Autodesk Inventor part; units mm, degrees
ref_plane "YZ Plane" through (0, 0, 0) normal (1, 0, 0) x (0, 1, 0)
ref_plane "XZ Plane" through (0, 0, 0) normal (0, 1, 0) x (-1, 0, 0)
ref_plane "XY Plane" through (0, 0, 0) normal (0, 0, 1) x (1, 0, 0)
sketch "Sketch1" plane through (0, 0, 0) normal (0, 1, 0) x (-1, 0, 0)
  line L0 (81, 0) -> (0, 0)
  line L1 (0, 0) -> (0, -32)
  line L2 (0, -32) -> (81, -32)
  line L3 (81, -32) -> (81, 0)
  point P0 (0, -16)
  point P1 (40.5, 0)
  dimension "d0" = 81
  dimension "d1" = 32
extrude "Extrusion1" add sketch "Sketch1" along normal blind 20
sketch "Sketch2" plane through (0, 0, 0) normal (1, 0, 0) x (0, 0, -1)
  line L0 (0, 0) -> (32, 0)
  line L1 (24.1, 0) -> (24.1, 6.35)
  line L2 (24.1, 6.35) -> (25.6, 6.35)
  line L3 (25.6, 6.35) -> (25.6, 9.525)
  line L4 (25.6, 9.525) -> (6.4, 9.525)
  line L5 (6.4, 9.525) -> (6.4, 6.35)
  line L6 (6.4, 6.35) -> (7.9, 6.35)
  line L7 (7.9, 6.35) -> (7.9, 0)
  line L8 (24.1, 0) -> (7.9, 0)
  line L9 (32, 0) -> (32, 20)
  line L10 (0, 0) -> (0, 20)
  dimension "d4" = 3.175
  dimension "d5" = 6.35
  dimension "d6" = 19.2
  dimension "d7" = 16.2
  dimension "d8" = 6.4
  dimension "d17" = 7.9
  dimension "d18" = 32
extrude "Extrusion2" cut sketch "Sketch2" against normal blind 103.1875
fillet "Fillet1" radius 2 1 edges at (-40.5, 20, -32)
fillet "Fillet2" radius 2 1 edges at (-40.5, 20, 0)
equation "\"d8\" = -0.5 * d6 + 0.5 * d18"
equation "\"d17\" = -0.5 * d7 + 0.5 * d18"
properties part number "rail holder"
Can you work these out from the model? Positions are in its coordinate system, mm. A direction names the side the tool comes from. Round coordinates to 2 decimals unless told otherwise and drop trailing zeros. Loops run counter-clockwise (first coordinate to the right, second up) from the corner with the lowest first, then second, coordinate; pieces in that order, holes last. Notation, with made-up numbers: M 13,67.25 L 23,67.25 A15 ccw 23,73.25 Z; hole C 68,27 d7. An arc over 180 degrees is marked long. Answer in a Markdown table with one row per item.
1. On a 3-axis mill with a long thin cutter (end or side, diameter ignored), from which of +Z, -Z, +X, -X, +Y, -Y can I reach the whole of each face in a straight line? I mean faces 1 (the face through (-40, 6.35, -7)), 2 (the face through (-40, 3, -7.9)), 3 (the face through (-41.07, 19.43, -31.4)). Say none if no direction works.
Established:
| item | result |
|---|---|
| face 1 | +X, -X |
| face 2 | +X, -X, -Y |
| face 3 | -Z, +X, -X, +Y |
2. If we section it at C-C, the plane z = -22: Please give me the cut outline in (x, y) (3 decimals).
Established:
| item | result |
|---|---|
| outline | M -81,9.525 L 0,9.525 L 0,20 L -81,20 Z |
3. Thinking about a two-plate mould opening in Y: for faces 4 (the face through (-40, 0, -4)), 5 (the face through (-40, 8, -6.4)), 6 (the face through (-41, 9, 0)), which applies, pulls with the +Y half, pulls with the -Y half, needs draft (parallel to the pull), parting line crosses it, or undercut?
Established:
| item | result |
|---|---|
| face 4 | pulls with the -Y half |
| face 5 | undercut |
| face 6 | needs draft |
4. If we section it at B-B, the plane x = -7: Please give me the cut outline in (y, z) (3 decimals), plus the area to 3 significant figures.
Established:
| item | result |
|---|---|
| outline | M 0,-32 L 18,-32 A2 ccw 20,-30 L 20,-2 A2 ccw 18,0 L 0,0 L 0,-7.9 L 6.35,-7.9 L 6.35,-6.4 L 9.525,-6.4 L 9.525,-25.6 L 6.35,-25.6 L 6.35,-24.1 L 0,-24.1 Z |
| area | 474 mm² |
5. If we section it at A-A, the plane y = 7.5: Please give me the cut outline in (x, z), plus the area to 3 significant figures.
Established:
| item | result |
|---|---|
| outline | M -81,-32 L 0,-32 L 0,-25.6 L -81,-25.6 Z; M -81,-6.4 L 0,-6.4 L 0,0 L -81,0 Z |
| area | 1,040 mm² |
6. Please list where these lines run through material, in increasing order: line 1 (Z direction, x = -4.5, y = 9); line 2 (Z direction, x = -34, y = 6); line 3 (Y direction, x = -11, z = -15) (3 decimals). Write a range as from..to.
Established:
| item | result |
|---|---|
| line 1 | -32..-25.6, -6.4..0 |
| line 2 | -32..-24.1, -7.9..0 |
| line 3 | 9.525..20 |
